Work out the finished part from the listing and answer in its coordinate system (mm). A direction names the side the tool comes from. Coordinates: 2 decimals unless noted, no trailing zeros. Loops run counter-clockwise (first coordinate to the right, second up) from the corner with the lowest first, then second, coordinate; pieces in that order, holes last. Notation, with made-up numbers: (72, 61.5) -> (101, 61.5) arc R21 cw to (101, 92.5) -> close; hole circle Ø11 at (47.25, 49). An arc over 180 degrees is marked (long way). Answer as CSV lines item,"result".
Autodesk Fusion 360 part; units mm, degrees
sketch "Esquisse1" plane through (0, 0, 0) normal (0, 0, 1) x (1, 0, 0)
  line L0 (0, 0) -> (44.5, 0)
  line L1 (49.2, 4.7) -> (49.2, 32.9)
  line L2 (44.5, 37.6) -> (0, 37.6)
  line L3 (0, 37.6) -> (0, 0)
  line L4 (0, 37.6) -> (-2, 37.6)
  line L5 (-2, 37.6) -> (-2, 0)
  line L6 (-2, 0) -> (0, 0)
  line L7 (0, 0) -> (0, 37.6)
  circle A0 centre (6.4, 34.4) radius 1.6
  circle A1 centre (6.4, 3.2) radius 1.6
  circle A2 centre (38.1, 34.4) radius 1.6
  circle A3 centre (44.5, 34.4) radius 1.6
  circle A4 centre (38.1, 3.2) radius 1.6
  circle A5 centre (44.5, 3.2) radius 1.6
  arc A6 (49.2, 32.9) -> (44.5, 37.6) centre (44.5, 32.9) ccw
  arc A7 (44.5, 0) -> (49.2, 4.7) centre (44.5, 4.7) ccw
  circle A8 centre (12.74, 3.2) radius 1.6
  circle A9 centre (19.08, 3.2) radius 1.6
  circle A10 centre (25.42, 3.2) radius 1.6
  circle A11 centre (31.76, 3.2) radius 1.6
  circle A12 centre (12.74, 34.4) radius 1.6
  circle A13 centre (19.08, 34.4) radius 1.6
  circle A14 centre (25.42, 34.4) radius 1.6
  circle A15 centre (31.76, 34.4) radius 1.6
  point P0 (49.2, 0)
  dimension "d1" = 49.2
  dimension "d2" = 37.6
  dimension "d3" = 2
  dimension "d6" = 3.2
  dimension "d7" = 8.4
  dimension "d8" = 3.2
  dimension "d10" = 3.2
  dimension "d11" = 3.2
  dimension "d12" = 8.4
  dimension "d19" = 3.2
  dimension "d20" = 3.2
  dimension "d25" = 3.2
  dimension "d26" = 3.2
  dimension "d27" = 4.7
  dimension "d28" = 4.7
  dimension "d29" = 6.4
  dimension "d30" = 6.4
  dimension "d31" = 4.7
  dimension "d32" = 4.7
  dimension "d48" = 3.2
  dimension "d49" = 3.2
  dimension "d50" = 3.2
  dimension "d51" = 3.2
  dimension "d52" = 3.2
  dimension "d53" = 3.2
  dimension "d54" = 3.2
  dimension "d55" = 3.2
extrude "Extrusion1" add sketch "Esquisse1" along normal blind 2 contours L0 L1 L2 L3 L7 A6 A7 | L3 L4 L5 L6 L7 | A0 | A1 | A2 | A3 | A4 | A5 | A8 | A9 | A10 | A11 | A12 | A13 | A14 | A15 makes body 1
extrude "Extrusion3" add sketch "Esquisse1" along normal blind 39.6 contours L3 L4 L5 L6 L7 bodies 1
sketch "Esquisse2" plane through (-2, 0, 0) normal (-1, 0, 0) x (0, -1, 0)
  line L0 (-37.6, 0) -> (0, 0)
  line L1 (0, 0) -> (0, 39.6)
  line L2 (0, 39.6) -> (-37.6, 39.6)
  line L3 (-37.6, 39.6) -> (-37.6, 0)
  circle A0 centre (-3.3, 20.8) radius 1.65
  circle A1 centre (-11.05, 34.2234) radius 1.65
  circle A2 centre (-26.55, 34.2234) radius 1.65
  circle A3 centre (-34.3, 20.8) radius 1.65
  circle A4 centre (-26.55, 7.3766) radius 1.65
  circle A5 centre (-11.05, 7.3766) radius 1.65
  line L4 (-25.4, 27.8) -> (-25.4, 13.8)
  line L5 (-12.2, 13.8) -> (-12.2, 27.8)
  line L6 (-12.2, 27.8) -> (-25.4, 13.8) construction
  line L7 (-25.4, 27.8) -> (-12.2, 13.8) construction
  arc A6 (-12.2, 27.8) -> (-25.4, 27.8) centre (-18.8, 27.8) ccw
  arc A7 (-25.4, 13.8) -> (-12.2, 13.8) centre (-18.8, 13.8) ccw
  arc A8 (-18.8, 39.6) -> (-37.6, 20.8) centre (-18.8, 20.8) ccw
  arc A9 (0, 20.8) -> (-18.8, 39.6) centre (-18.8, 20.8) ccw
  point P0 (-18.8, 20.8)
  dimension "d39" = 3.3
  dimension "d42" = 13.2
  dimension "d43" = 14
extrude "Extrusion4" cut sketch "Esquisse2" against normal blind 19 contours A0 | A1 | A2 | A3 | A4 | A5 | L4 L5 A6 A7 bodies 1
extrude "Extrusion5" cut sketch "Esquisse1" along normal blind 8 contours A0 | A1 | A2 | A3 | A4 | A5 | A8 | A9 | A10 | A11 | A12 | A13 | A14 | A15 bodies 1
copy_body "Corps->Comp3" bodies 1 removing the originals makes body 2 in component "Component"
component "Component" placed x (1, 0, 0) y (0, 1, 0) z (0, 0, 1) at (0, 0, 0)
(1) Flat-ended cylindrical pins translate along their axes: pin 1 Ø12 at (y, z) = (18, 35) entering from +X; pin 2 Ø6 at (x, y) = (13.5, 25.5) entering from +Z. Find the tip coordinate at first contact, or state that the pin passes through.
Computed values:
pin 1,"x = 0"
pin 2,"z = 2"
(2) A cutting plane is placed at C-C, the plane z = 25.5. Write down the section's boundary in (x, y).
Computed values:
outline,"(-2, 0) -> (0, 0) -> (0, 12.2) -> (-2, 12.2) -> close; (-2, 25.4) -> (0, 25.4) -> (0, 37.6) -> (-2, 37.6) -> close"
(3) A cutting plane is placed at A-A, the plane x = 25.42. Write down the section's boundary in (y, z).
Computed values:
outline,"(0, 0) -> (1.6, 0) -> (1.6, 2) -> (0, 2) -> close; (4.8, 0) -> (32.8, 0) -> (32.8, 2) -> (4.8, 2) -> close; (36, 0) -> (37.6, 0) -> (37.6, 2) -> (36, 2) -> close"
(4) Consider line 1 along Z through (x, y) = (-0.75, 11.05); line 2 along Y through (x, z) = (19.08, 1.5); line 3 along Z through (x, y) = (9, 25.5). Determine where each line is inside the solid, lowest interval first.
Computed values:
line 1,"0 to 5.73, 9.03 to 32.57, 35.87 to 39.6"
line 2,"0 to 1.6, 4.8 to 32.8, 36 to 37.6"
line 3,"0 to 2"
(5) Which of the six approach directions +Z, -Z, +X, -X, +Y, -Y give full straight-line access (tool end or side, diameter ignored) to faces 4 (the face through (0, 27, 21)), 5 (the face through (-1, 18.9, 7.2)), 6 (the face through (36.92, 2.12, 0.99))?
Computed values:
face 4,"+Z, +X, +Y, -Y"
face 5,"+X, -X"
face 6,"+Z, -Z"
(6) A cutting plane is placed at D-D, the plane y = 18.8. Write down the section's boundary in (x, z), and give its area (3 significant figures).
Computed values:
outline,"(-2, 0) -> (49.2, 0) -> (49.2, 2) -> (0, 2) -> (0, 7.2) -> (-2, 7.2) -> close; (-2, 34.4) -> (0, 34.4) -> (0, 39.6) -> (-2, 39.6) -> close"
area,"123 mm2"
(7) A cutting plane is placed at B-B, the plane y = 26.55. Write down the section's boundary in (x, z).
Computed values:
outline,"(-2, 0) -> (49.2, 0) -> (49.2, 2) -> (0, 2) -> (0, 5.73) -> (-2, 5.73) -> close; (-2, 9.03) -> (0, 9.03) -> (0, 32.57) -> (-2, 32.57) -> close; (-2, 35.87) -> (0, 35.87) -> (0, 39.6) -> (-2, 39.6) -> close"
(8) For a pull along Y with two mould halves and no side action, classify faces 1 (the face through (24, 19, 2)), 2 (the face through (11, 37.6, 1)), 3 (the face through (-1.01, 27.86, 33.22)) as pulls with the +Y half, pulls with the -Y half, needs draft (parallel to the pull), parting line crosses it, or undercut.
Computed values:
face 1,"needs draft"
face 2,"pulls with the +Y half"
face 3,"undercut"
